from build123d import *

# Parameters (mm, degrees)
BOSS_EXTRUDE1_DEPTH = 20
SKETCH2_R           = 2.25
CUT_EXTRUDE1_DEPTH  = 20
SKETCH3_R           = 1.5
CUT_EXTRUDE2_DEPTH  = 20
FILLET1_R           = 1
FILLET2_R           = 1


with BuildPart() as part:
    # Sketch1 → Boss-Extrude1 (new body)
    with BuildSketch(Plane.XY):
        Polygon((0, -10.581899729), (0, 12.318100271), (-7, 12.318100271), (-7, 15.318100271), (3, 15.318100271), (3, -13.581899729), (-7, -13.581899729), (-7, -10.581899729), align=None)
    extrude(amount=BOSS_EXTRUDE1_DEPTH)

    # Sketch2 → Cut-Extrude1 (cut)
    with BuildSketch(Plane(origin=(0, 15.318100271, 0), x_dir=(1, 0, 0), z_dir=(0, 1, 0))):
        with Locations((-1, -5)):
            Circle(SKETCH2_R)
        with Locations((-1, -15)):
            Circle(SKETCH2_R)
    extrude(amount=-CUT_EXTRUDE1_DEPTH, mode=Mode.SUBTRACT)

    # Sketch3 → Cut-Extrude2 (cut)
    with BuildSketch(Plane(origin=(0, -10.581899729, 0), x_dir=(1, 0, 0), z_dir=(0, 1, 0))):
        with Locations((-3.5, -4)):
            Circle(SKETCH3_R)
        with Locations((-3.5, -10)):
            Circle(SKETCH3_R)
        with Locations((-3.5, -16)):
            Circle(SKETCH3_R)
    extrude(amount=-CUT_EXTRUDE2_DEPTH, mode=Mode.SUBTRACT)

    # Fillet1
    fillet1_edges = [part.edges().sort_by_distance(p)[0] for p in [
        (-7, -12.081899729, 0),
        (0, -10.581899729, 10),
        (-7, 12.318100271, 10),
        (-7, 13.818100271, 20),
        (-7, -12.081899729, 20),
        (-7, 13.818100271, 0),
    ]]
    fillet(fillet1_edges, radius=FILLET1_R)

    # Fillet2
    fillet2_edges = [part.edges().sort_by_distance(p)[0] for p in [
        (0, 12.318100271, 18.507782219),
        (0, 12.318100271, 10),
        (0, 12.318100271, 1.492217781),
    ]]
    fillet(fillet2_edges, radius=FILLET2_R)


solid = part.part
Verification items for the finished model (mm, model axes). A direction names the side the tool comes from. Coordinates: 2 decimals unless noted, no trailing zeros. Order: outer loops, then holes, each group sorted by start corner. A loop starts at its lowest first (then second) coordinate and runs counter-clockwise, first axis right, second up. Notation, with made-up numbers: M -33.5,23.25 L -7.5,23.25 A30 cw -7.5,51.25 Z; hole C 81,10 d7. An arc over 180 degrees is marked long. One line per item, written item: value. Start each with the question number.
Item 1: Access from +Z, -Z, +X, -X, +Y, -Y to the whole of each face (thin tool, end or side, straight path). Record for faces 1 (the flat face through (0.5, -4.682, 15)), 2 (the cylindrical face through (-2.81, -12.06, 11.33)), 3 (the cylindrical face through (-6.699, 12.603, 10.14)), 4 (the cylindrical face through (-6.699, -12.061, 19.715)), 5 (the cylindrical face through (1.08, 5.46, 5.86)).
Item 2: Sectioned sample at B-B on y = 10.75. Record the cut outline in (x, z), then the cut area to 3 significant figures.
Item 3: Sectioned sample at C-C on z = 16. Record the cut outline in (x, y), then the cut area to 3 significant figures.
Item 4: Thickness scan on probe 1 along Z at (x, y) = (-3.5, -12.25); probe 2 along Y at (x, z) = (-4.25, 5.5); probe 3 along X at (y, z) = (-11.25, 4). Record the ranges inside material, lowest first.
Item 5: Sectioned sample at D-D on x = 0.5. Record the cut outline in (y, z).
Item 6: Depth check by flat-ended pin: P1, Ø8, axis at y = 11, z = 12.5, coming from the -X side; P2, Ø1, axis at y = -2.5, z = 11, coming from the -X side; P3, Ø1.8, axis at x = -3.5, z = 4, coming from the -Y side; P4, Ø3.5, axis at x = -1, z = 5, coming from the +Y side. Enter the tip coordinate at first touch or a pass-through.
Item 7: Sectioned sample at A-A on z = 10. Record the cut outline in (x, y).
Item 8: Mould release check, pull along X, two halves, no side actions. Record for faces 6 (the cylindrical face through (-2, -12, 4)), 7 (the flat face through (3, 1, 10)), 8 (the flat face through (-4, 12.318, 10)): pulls with the +X half, pulls with the -X half, needs draft (parallel to the pull), parting line crosses it, or undercut.
Calculated:
1. face 1: -X, +Y
1. face 2: -Y
1. face 3: +Z, -Z, -X
1. face 4: +Z, -X, +Y, -Y
1. face 5: +Y
2. outline: M 0,0 L 3,0 L 3,20 L 0,20 L 0,17.02 A2.25 cw 0,12.98 L 0,7.02 A2.25 cw 0,2.98 Z
2. area: 52.8 mm^2
3. outline: M -7,-13.58 L -5,-13.58 L -5,-10.58 L -7,-10.58 Z; M -7,13.32 A1 ccw -6,12.32 L -3.02,12.32 L -3.02,15.32 L -7,15.32 Z; M -2,-13.58 L 3,-13.58 L 3,15.32 L 1.02,15.32 L 1.02,-4.68 L 0,-4.68 L 0,-9.58 A1 cw -1,-10.58 L -2,-10.58 Z
3. area: 90.3 mm^2
4. probe 1: 0 to 2.5, 5.5 to 8.5, 11.5 to 14.5, 17.5 to 20
4. probe 2: -13.58 to -10.58, 12.32 to 15.32
4. probe 3: -7 to -5, -2 to 3
5. outline: M -13.58,0 L 15.32,0 L 15.32,3.32 L -4.68,3.32 L -4.68,6.68 L 15.32,6.68 L 15.32,13.32 L -4.68,13.32 L -4.68,16.68 L 15.32,16.68 L 15.32,20 L -13.58,20 Z
6. P1: x = -7
6. P2: x = 0
6. P3: y = 12.32
6. P4: y = -4.68
7. outline: M -7,-13.58 L -5,-13.58 L -5,-10.58 L -7,-10.58 Z; M -7,13.32 A1 ccw -6,12.32 L -1,12.32 A1 cw 0,11.32 L 0,-9.58 A1 cw -1,-10.58 L -2,-10.58 L -2,-13.58 L 3,-13.58 L 3,15.32 L -7,15.32 Z
8. face 6: undercut
8. face 7: pulls with the +X half
8. face 8: needs draft
